Read the model definition and answer for the solid it produces. Units are mm, in the model's axes. Give positions to 0.01 mm unless a question says otherwise; leave off trailing zeros. Order: outer loops, then holes, each group sorted by start corner. A loop starts at its lowest first (then second) coordinate and runs counter-clockwise, first axis right, second up. Notation, with made-up numbers: (52, 48) - (77, 48) arc R20 cw to (77, 81) - close; hole circle Ø5 at (78.5, -9). An arc over 180 degrees is marked (long way). Answer as CSV lines item,"result". Start each with the question number.
from build123d import *

# Parameters (mm, degrees)
SKETCH_W     = 110
SKETCH_H     = 80
PAD_DEPTH    = 2
SKETCH001_R  = 2.1
POCKET_DEPTH = 5
CHAMFER_SIZE = 1


with BuildPart() as part:
    # Sketch → Pad (new body)
    with BuildSketch(Plane.XY):
        Rectangle(SKETCH_W, SKETCH_H)
    extrude(amount=PAD_DEPTH)

    # Sketch001 (on Face6 of Pad) → Pocket (cut)
    with BuildSketch(Plane.XY.offset(2)):
        with Locations((49, 34)):
            Circle(SKETCH001_R)
        with Locations((-49, 34)):
            Circle(SKETCH001_R)
        with Locations((-49, -34)):
            Circle(SKETCH001_R)
        with Locations((49, -34)):
            Circle(SKETCH001_R)
    extrude(amount=-POCKET_DEPTH, mode=Mode.SUBTRACT)

    # Chamfer
    chamfer_edges = [part.edges().sort_by_distance(p)[0] for p in [
        (-51.1, -34, 0),
        (-51.1, 34, 0),
        (46.9, 34, 0),
        (46.9, -34, 0),
    ]]
    chamfer(chamfer_edges, length=CHAMFER_SIZE)


solid = part.part
(1) A straight line is drawn through the part: line 1 (Y direction, x = -49, z = 1.5). Find the intervals that lie inside material, in ascending order. Write a range as [from, to].
(2) A flat-ended cylindrical pin translates along its axis: pin 1 Ø8 at (x, y) = (33.5, -3.5) entering from -Z. Find the tip coordinate at first contact, or state that the pin passes through.
(3) Section B-B, the plane y = 34 is taken. Write down the section's boundary in (x, z), and give its area (3 significant figures).
(4) Section A-A, the plane x = -49 is taken. Write down the section's boundary in (y, z).
(5) Determine the mould class of faces 1 (the cylindrical face through (49.969, 32.137, 1.507)), 2 (the flat face through (-1, 1, 2)) for opening direction X: released by +X, released by -X, zero draft, split by the parting line, or undercut.
Checks:
1,line 1,"y = [-40, -36.1], [-31.9, 31.9], [36.1, 40]"
2,pin 1,"stops at z = 0"
3,outline,"(-55, 0) - (-52.1, 0) - (-51.1, 1) - (-51.1, 2) - (-55, 2) - close; (-46.9, 1) - (-45.9, 0) - (45.9, 0) - (46.9, 1) - (46.9, 2) - (-46.9, 2) - close; (51.1, 1) - (52.1, 0) - (55, 0) - (55, 2) - (51.1, 2) - close"
3,area,"201 mm²"
4,outline,"(-40, 0) - (-37.1, 0) - (-36.1, 1) - (-36.1, 2) - (-40, 2) - close; (-31.9, 1) - (-30.9, 0) - (30.9, 0) - (31.9, 1) - (31.9, 2) - (-31.9, 2) - close; (36.1, 1) - (37.1, 0) - (40, 0) - (40, 2) - (36.1, 2) - close"
5,face 1,"undercut"
5,face 2,"zero draft"
